```python
from build123d import *

# Parameters (mm, degrees)
SKETCH_1_W          = 20.5
SKETCH_1_H          = 40.5
SKETCH_1_W_2        = 25
SKETCH_1_H_2        = 12.5
SKETCH_1_W_3        = 14
SKETCH_1_H_3        = 7
EXTRUDE_1367_DEPTH  = 3
FILLET_1_R          = 10
FILLET_2_R          = 1.5
HOLE_WIZARD_3_5_D   = 3.5
HOLE_WIZARD_3_5_2_D = 3.5


with BuildPart() as part:
    # Эскиз1 → Extrude 1367 (new, symmetric)
    with BuildSketch(Plane(origin=(0, 0, 0), x_dir=(1, 0, 0), z_dir=(0, 1, 0))):
        Polygon((273.664027596, -136.63804004), (18.5, 305.31902002), (-18.5, 305.31902002), (-273.664027596, -136.63804004), (-255.164027596, -168.68097998), (255.164027596, -168.68097998), align=None)
        Polygon((219.01884632, -138.286270399), (254.092875173, -158.536270399), (264.342875173, -140.782749621), (229.26884632, -120.532749621), align=None, mode=Mode.SUBTRACT)
        with Locations((0, 279.06902002)):
            Rectangle(SKETCH_1_W, SKETCH_1_H, mode=Mode.SUBTRACT)
        Polygon((-229.26884632, -120.532749621), (-264.342875173, -140.782749621), (-254.092875173, -158.536270399), (-219.01884632, -138.286270399), align=None, mode=Mode.SUBTRACT)
        Polygon((216.537439859, -110.584192463), (204.037439859, -132.234827557), (193.212122312, -125.984827557), (205.712122312, -104.334192463), align=None, mode=Mode.SUBTRACT)
        with Locations((0, 236.56902002)):
            Rectangle(SKETCH_1_W_2, SKETCH_1_H_2, mode=Mode.SUBTRACT)
        Polygon((-204.037439859, -132.234827557), (-216.537439859, -110.584192463), (-205.712122312, -104.334192463), (-193.212122312, -125.984827557), align=None, mode=Mode.SUBTRACT)
        with Locations((0, 136.5)):
            Rectangle(SKETCH_1_W_3, SKETCH_1_H_3, mode=Mode.SUBTRACT)
    extrude(amount=EXTRUDE_1367_DEPTH, both=True)

    # Скругление1
    fillet_1_edges = [part.edges().sort_by_distance(p)[0] for p in [
        (255.164027596, 0, 168.68097998),
        (-255.164027596, 0, 168.68097998),
        (-273.664027596, 0, 136.63804004),
        (-18.5, 0, -305.31902002),
        (18.5, 0, -305.31902002),
        (273.664027596, 0, 136.63804004),
    ]]
    fillet(fillet_1_edges, radius=FILLET_1_R)

    # Скругление2
    fillet_2_edges = [part.edges().sort_by_distance(p)[0] for p in [
        (10.25, 0, -258.81902002),
        (10.25, 0, -299.31902002),
        (-10.25, 0, -299.31902002),
        (-10.25, 0, -258.81902002),
        (12.5, 0, -230.31902002),
        (12.5, 0, -242.81902002),
        (-12.5, 0, -242.81902002),
        (-12.5, 0, -230.31902002),
        (229.26884632, 0, 120.532749621),
        (219.01884632, 0, 138.286270399),
        (254.092875173, 0, 158.536270399),
        (264.342875173, 0, 140.782749621),
        (-219.01884632, 0, 138.286270399),
        (-229.26884632, 0, 120.532749621),
        (-264.342875173, 0, 140.782749621),
        (-254.092875173, 0, 158.536270399),
        (-7, 0, -140),
        (-7, 0, -133),
        (7, 0, -133),
        (7, 0, -140),
        (193.212122312, 0, 125.984827557),
        (204.037439859, 0, 132.234827557),
        (216.537439859, 0, 110.584192463),
        (205.712122312, 0, 104.334192463),
        (-205.712122312, 0, 104.334192463),
        (-216.537439859, 0, 110.584192463),
        (-204.037439859, 0, 132.234827557),
        (-193.212122312, 0, 125.984827557),
    ]]
    fillet(fillet_2_edges, radius=FILLET_2_R)

    # Hole Wizard 3_5 (through all)
    with Locations(Plane.XZ.offset(3)):
        with Locations((-100, 127.305734356), (-160.25, 22.9496732), (100, 127.305734356), (160.25, 22.9496732), (-60.25, -150.255407557), (60.25, -150.255407557)):
            Hole(HOLE_WIZARD_3_5_D / 2)

    # Hole Wizard 3_5 2 (through all)
    with Locations(Plane(origin=(0, 3, 0), x_dir=(1, 0, 0), z_dir=(0, 1, 0))):
        with Locations((-137.42175976, 79.34048999), (-62.42175976, 209.244300558), (62.42175976, 209.244300558), (137.42175976, 79.34048999), (212.42175976, -50.563320578), (150, -158.68097998), (0, -158.68097998), (-150, -158.68097998), (-212.42175976, -50.563320578)):
            Hole(HOLE_WIZARD_3_5_2_D / 2)


solid = part.part
```
Work out the finished part from the listing and answer in its coordinate system (mm). A direction names the side the tool comes from. Coordinates: 2 decimals unless noted, no trailing zeros. Order: outer loops, then holes, each group sorted by start corner. A loop starts at its lowest first (then second) coordinate and runs counter-clockwise, first axis right, second up. Notation, with made-up numbers: M 6,-3 L 64,-3 A16 ccw 64,10 Z; hole C -13,17.5 d7. An arc over 180 degrees is marked long. Use CSV: the item, a comma, the result in double quotes.
1) Flat-ended cylindrical pins translate along their axes: pin 1 Ø2 at (y, z) = (0, -136) entering from +X; pin 2 Ø1 at (x, y) = (110, -1) entering from -Z; pin 3 Ø1.8 at (y, z) = (-1, -280) entering from -X. Find the tip coordinate at first contact, or state that the pin passes through.
Worked out:
pin 1,"stops at x = 116.83"
pin 2,"stops at z = -147.7"
pin 3,"stops at x = -33.64"
2) Section A-A on z = -272 is taken. Write down the section's boundary in (x, y).
Worked out:
outline,"M -37.74,-3 L -10.25,-3 L -10.25,3 L -37.74,3 Z; M 10.25,-3 L 37.74,-3 L 37.74,3 L 10.25,3 Z"
3) Consider line 1 (Z direction, x = 100, y = 0.6); line 2 (Z direction, x = 236.5, y = -2.65); line 3 (Z direction, x = -72, y = -0.5). Determine where each line is inside the solid, lowest interval first. Write a range as [from, to].
Worked out:
line 1,"z = [-164.16, 125.56], [129.06, 168.68]"
line 2,"z = [72.27, 124.71], [148.38, 168.68]"
line 3,"z = [-212.65, 168.68]"
4) Determine the mould class of faces 1 (the face through (-264.5, 0.04, 152.51)), 2 (the face through (-246.579, 0.042, 130.526)), 3 (the face through (147.828, 0.042, -81.317)) for opening direction Z: released by +Z, released by -Z, zero draft, split by the parting line, or undercut.
Worked out:
face 1,"released by +Z"
face 2,"undercut"
face 3,"released by -Z"
5) Section C-C on x = 47 is taken. Write down the section's boundary in (y, z), plus the area to 3 significant figures.
Worked out:
outline,"M -3,-255.96 L 3,-255.96 L 3,168.68 L -3,168.68 Z"
area,"2,550 mm^2"
6) For faces 4 (the face through (236.33, 0.04, 148.28)), 5 (the face through (-4, 3, -19)), determine the directions among +Z, -Z, +X, -X, +Y, -Y from which every point of the face is accessible in a straight line to the end or side of a thin tool.
Worked out:
face 4,"+Y, -Y"
face 5,"+Z, -Z, +X, -X, +Y"
7) Section D-D on x = -42 is taken. Write down the section's boundary in (y, z).
Worked out:
outline,"M -3,-264.62 L 3,-264.62 L 3,168.68 L -3,168.68 Z"
8) Section B-B on y = 0.85 is taken. Count the separate pieces of the cut face and the enclosed holes in it, plus the area to 3 significant figures.
Worked out:
separate pieces,"1"
enclosed holes,"22"
area,"142,000 mm^2"
